Design review of the part shown in the three views and the two pictorial views. Dimensions are in mm from the part's minimum x, y and z. A direction names the side the tool comes from. Give positions to 0.01 mm unless a question says otherwise; leave off trailing zeros. Order: outer loops, then holes, each group sorted by start corner. A loop starts at its lowest first (then second) coordinate and runs counter-clockwise, first axis right, second up. Notation, with made-up numbers: M 50.5,73.25 L 87.5,73.25 A8 cw 87.5,88.25 Z; hole C 13.25,-36 d3. An arc over 180 degrees is marked long. Answer as a JSON object with one key per item and string values.
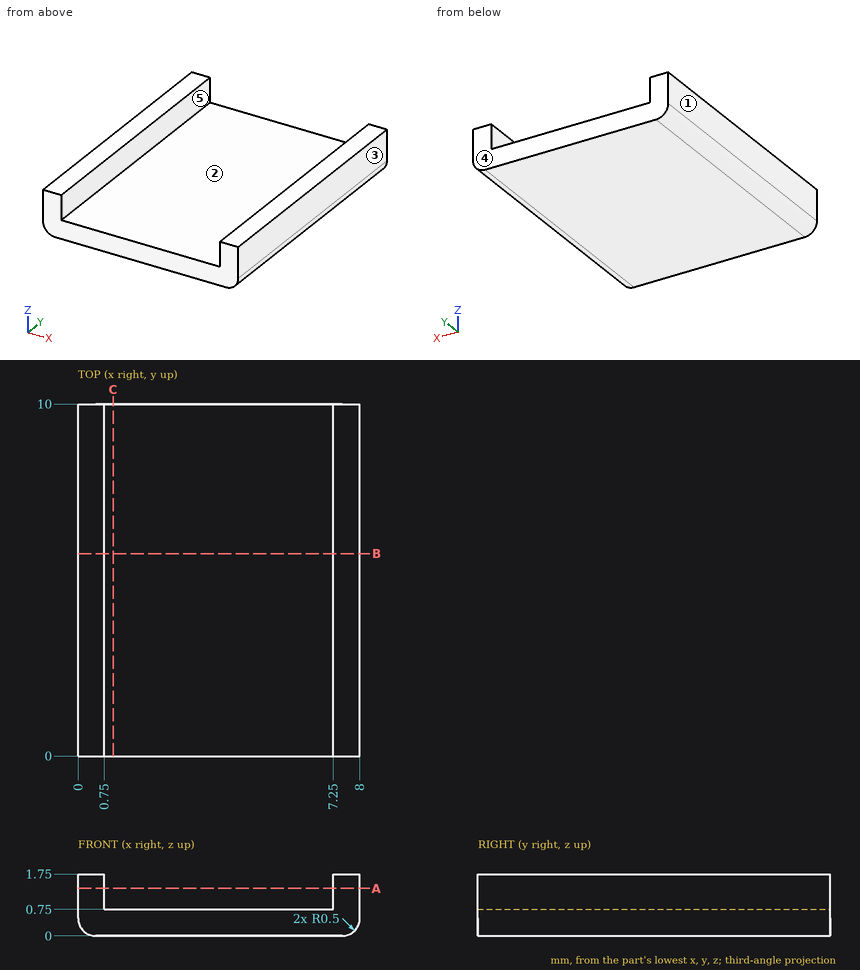
(1) Draft analysis for pull direction X (two halves, no side actions). For the marked faces 1, 2 and 3, state which applies: +X half, -X half, draft (parallel to the pull), parting line (faces both ways), or undercut.
Checked values:
{"face 1": "-X half", "face 2": "undercut", "face 3": "+X half"}
(2) We need section C-C (x = 1). Write out the cut boundary in (y, z).
Checked values:
{"outline": "M 0,0 L 10,0 L 10,0.75 L 0,0.75 Z"}
(3) Tool access review of the marked faces 4 and 5: name each direction out of +Z, -Z, +X, -X, +Y, -Y from which nothing blocks a thin tool from reaching the whole face with its end or side.
Checked values:
{"face 4": "+Z, -Z, +X, -X, +Y", "face 5": "+Z, +Y, -Y"}
(4) We need section B-B (y = 5.75). Write out the cut boundary in (x, z).
Checked values:
{"outline": "M 0,0.5 A0.5 ccw 0.5,0 L 7.5,0 A0.5 ccw 8,0.5 L 8,1.75 L 7.25,1.75 L 7.25,0.75 L 0.75,0.75 L 0.75,1.75 L 0,1.75 Z"}
(5) We need section A-A (z = 1.35). Write out the cut boundary in (x, y), plus the area to 3 significant figures.
Checked values:
{"outline": "M 0,0 L 0.75,0 L 0.75,10 L 0,10 Z; M 7.25,0 L 8,0 L 8,10 L 7.25,10 Z", "area": "15.0 mm^2"}
(6) To check wall thickness, follow L1, parallel to X at y = 4.5, z = 1; L2, parallel to Z at x = 6.5, y = 8; L3, parallel to Z at x = 7.75, y = 5.75. State the ranges of each line that lie inside material, in increasing order. Write a range as from..to.
Checked values:
{"L1": "x = 0..0.75, 7.25..8", "L2": "z = 0..0.75", "L3": "z = 0.07..1.75"}
(7) Insertion check: pin 1 (1 mm diameter, centred on x = 4.5, y = 3, fed in from +Z). The pin has a flat end and moves straight along its axis. Give the tip position at first contact, or say it passes through.
Checked values:
{"pin 1": "stops at z = 0.75"}
